Geometry: final body of the model. Coordinates: model frame, mm. A direction names the side the tool comes from. Give positions to 0.01 mm unless a question says otherwise; leave off trailing zeros. Order: outer loops, then holes, each group sorted by start corner. A loop starts at its lowest first (then second) coordinate and runs counter-clockwise, first axis right, second up. Notation, with made-up numbers: (1, -1) -> (40, -1) arc R21 ccw to (40, 28) -> close; hole circle Ø7 at (79.5, 32). An arc over 180 degrees is marked (long way). Answer in a Markdown table with one row per item. Add a question column.
Q1. Line query: line 1 along X through (y, z) = (20.5, -10.5); line 2 along Z through (x, y) = (-19, 11); line 3 along Y through (x, z) = (31, -78). Output: solid intervals per line, ascending. Write a range as from..to.
Q2. Set-up query: faces 1 (the face through (-99, 29.8, -10)), 2 (the face through (104, 20, -20)), 3 (the face through (-35.621, 5.029, -60.857)), 4 (the face through (1.92, 45.63, -87.48)), 5 (the face through (-104, 20, -20)). Return all of +Z, -Z, +X, -X, +Y, -Y with unobstructed straight access to the full face (end or side cutting, diameter ignored); none if empty.
Q3. Cut plane A-A on y = -11.5. Return the cut outline in (x, z), and give its area (3 significant figures).
Q4. Pull-direction query (Z, two-part tool) for faces 6 (the face through (-97, 64.8, -26)), 7 (the face through (99, 9.8, -10)), 8 (the face through (47.145, 1.496, -37.58)); classes: +Z half, -Z half, draft (parallel to the pull), parting line (faces both ways), or undercut.
Q5. Contact query for flat-ended pins moving along their axis: P1, Ø2, axis at x = -18.5, z = -18.5, coming from the -Y side; P2, Ø8, axis at y = -9, z = -77.5, coming from the -X side; P3, Ø4.5, axis at x = -96, z = -23, coming from the -Y side; P4, Ø3, axis at x = 46, y = 32.5, coming from the -Z side. Output: stop coordinate, or through.
from build123d import *
from build123d.topology import SkipClean

# Parameters (mm, degrees)
REVOLU_O2_ANGLE                     = 180
ESBO_O4_R                           = 10
RESSALTO_EXTRUS_O1_DEPTH            = 35
RESSALTO_EXTRUS_O2_DEPTH            = 20
ESBO_O6_R                           = 2.5
CORTE_EXTRUS_O1_DEPTH               = 15
ESBO_O9_R                           = 1.25
CORTE_EXTRUS_O3_DEPTH               = 6
RESSALTO_EXTRUS_O6_DEPTH            = 20
RESSALTO_EXTRUS_O7_DEPTH            = 20
CORTE_EXTRUS_O6_START               = 10
ESBO_O16_R                          = 93
CORTE_EXTRUS_O6_DEPTH               = 10
PADR_OCIRCULAR1_COUNT               = 2
PADR_OCIRCULAR1_ANGLE               = 60
PADR_OCIRCULAR1_THE_OTHER_WAY_COUNT = 2
PADR_OCIRCULAR1_THE_OTHER_WAY_ANGLE = 60
ESBO_O46_R                          = 3
CORTE_EXTRUS_O14_DEPTH              = 30
CORTE_EXTRUS_O15_DEPTH              = 175.966168158
CORTE_EXTRUS_O15_DEPTH_BACK         = 175.966168158


with BuildPart() as part:
    # Esboço3 → Revolução2 (revolve)
    with BuildSketch(Plane.XY):
        with BuildLine():
            Line((97.5, 79.8), (97.5, 11.304491341))
            Line((97.5, 11.304491341), (97.5, 0))
            Line((97.5, 0), (97.5, -40.2))
            Line((97.5, -40.2), (79.5, -40.2))
            Line((79.5, -40.2), (79.5, 0))
            Line((79.5, 0), (60.342408243, 0))
            Line((60.342408243, 0), (60.239391973, 2.95))
            Line((60.239391973, 2.95), (52, 2.95))
            Line((52, 2.95), (44, 10.95))
            Line((44, 10.95), (31, 10.95))
            Line((31, 10.95), (31, 13.7))
            Line((31, 13.7), (22.6, 13.7))
            Line((22.6, 13.7), (22.6, 17))
            Line((22.6, 17), (19.3, 17))
            Line((19.3, 17), (19.3, 17.7))
            Line((19.3, 17.7), (15.3, 17.7))
            Line((15.3, 17.7), (15.3, 21.05))
            Line((15.3, 21.05), (19.3, 21.05))
            Line((19.3, 21.05), (19.3, 21.2))
            Line((19.3, 21.2), (27.626549127, 25.96))
            Line((27.626549127, 25.96), (31.3, 25.96))
            Line((31.3, 25.96), (31.3, 43.96))
            Line((31.3, 43.96), (32.3, 44.96))
            Line((32.3, 44.96), (38.8, 44.96))
            Line((38.8, 44.96), (38.8, 26.9))
            Line((38.8, 26.9), (55.5, 10.2))
            Line((55.5, 10.2), (83.5, 10.2))
            ThreePointArc((83.5, 10.2), (86.328427125, 11.371572875), (87.5, 14.2))
            Line((87.5, 14.2), (87.5, 76.2))
            Line((87.5, 76.2), (93, 76.2))
            Line((93, 76.2), (93, 79.8))
            Line((93, 79.8), (97.5, 79.8))
        make_face()
    revolve(axis=Axis((0, -3.322055656, 0), (0, 1, 0)), revolution_arc=REVOLU_O2_ANGLE)

    # Esboço20 → Revolução3 (revolve)
    with SkipClean():  # the faces are left unmerged after this step: merging them gives an invalid solid
        with BuildSketch(Plane.XY, mode=Mode.PRIVATE) as revolu_o3_sk:
            Polygon((60.342408243, 2.95), (60.342408243, 10.2), (55.5, 10.2), (38.8, 26.9), (38.8, 44.96), (32.3, 44.96), (31.3, 43.96), (31.3, 25.96), (27.626549127, 25.96), (19.3, 21.2), (19.3, 21.05), (15.3, 21.05), (15.3, 17.7), (19.3, 17.7), (19.3, 17), (22.6, 17), (22.6, 13.7), (31, 13.7), (31, 10.95), (44, 10.95), (52, 2.95), align=None)
        revolve(revolu_o3_sk.sketch.rotate(Axis((0, -3.322055656, 0), (0, 1, 0)), 90), axis=Axis((0, -3.322055656, 0), (0, 1, 0)))
    add(part.part.scale(1), mode=Mode.REPLACE)  # the faces are merged on a copy

    # Esboço4 → Ressalto-extrusão1 (add)
    with BuildSketch(Plane(origin=(0, 79.8, 0), x_dir=(1, 0, 0), z_dir=(0, 1, 0))):
        with Locations((25.881656302, 96.591656302)):
            Circle(ESBO_O4_R)
        with Locations((-96.591656302, 25.881656302)):
            Circle(ESBO_O4_R)
    extrude(amount=-RESSALTO_EXTRUS_O1_DEPTH)

    # Esboço5 → Ressalto-extrusão2 (add)
    with BuildSketch(Plane.XZ.offset(40.2)):
        with BuildLine():
            Line((10, -105), (10, -96.985823706))
            Line((10, -96.985823706), (-10, -96.985823706))
            Line((-10, -96.985823706), (-10, -105))
            ThreePointArc((-10, -105), (0, -115), (10, -105))
        make_face()
    ressalto_extrus_o2 = extrude(amount=-RESSALTO_EXTRUS_O2_DEPTH)

    # Esboço6 → Corte-extrusão1 (cut)
    with BuildSketch(Plane(origin=(0, 79.8, 0), x_dir=(1, 0, 0), z_dir=(0, 1, 0))):
        with Locations(Location((25.881656302, 96.591656302, 0), (0, 0, 270))):
            Circle(ESBO_O6_R)
        with Locations(Location((-96.591656302, 25.881656302, 0), (0, 0, 270))):
            Circle(ESBO_O6_R)
    extrude(amount=-CORTE_EXTRUS_O1_DEPTH, mode=Mode.SUBTRACT)

    # Esboço9 → Corte-extrusão3 (cut)
    with BuildSketch(Plane.XZ.offset(-13.7)):
        with Locations(Location((18.738329701, -18.738329701, 0), (0, 0, 270))):
            Circle(ESBO_O9_R)
        with Locations(Location((-18.738329701, -18.738329701, 0), (0, 0, 270))):
            Circle(ESBO_O9_R)
        with Locations(Location((-18.738329701, 18.738329701, 0), (0, 0, 270))):
            Circle(ESBO_O9_R)
        with Locations(Location((18.738329701, 18.738329701, 0), (0, 0, 270))):
            Circle(ESBO_O9_R)
    extrude(amount=-CORTE_EXTRUS_O3_DEPTH, mode=Mode.SUBTRACT)

    # Esboço12 → Ressalto-extrusão6 (add)
    with BuildSketch(Plane.XY):
        with BuildLine():
            Line((-102, 29.8), (-87.5, 29.8))
            Line((-87.5, 29.8), (-87.5, 9.8))
            Line((-87.5, 9.8), (-102, 9.8))
            ThreePointArc((-102, 9.8), (-112, 19.8), (-102, 29.8))
        make_face()
    extrude(amount=-RESSALTO_EXTRUS_O6_DEPTH)

    # Esboço13 → Ressalto-extrusão7 (add)
    with BuildSketch(Plane.XY):
        with BuildLine():
            Line((102, 29.8), (93.1, 29.8))
            Line((93.1, 29.8), (93.1, 9.8))
            Line((93.1, 9.8), (102, 9.8))
            ThreePointArc((102, 9.8), (112, 19.8), (102, 29.8))
        make_face()
    extrude(amount=-RESSALTO_EXTRUS_O7_DEPTH)

    # Esboço16 → Corte-extrusão6 (cut)
    with BuildSketch(Plane(origin=(0, 76.2, 0), x_dir=(1, 0, 0), z_dir=(0, 1, 0)).offset(CORTE_EXTRUS_O6_START)):
        Circle(ESBO_O16_R)
    extrude(amount=-CORTE_EXTRUS_O6_DEPTH, mode=Mode.SUBTRACT)

    # PadrãoCircular1: Ressalto-extrusão2 ×2 about axis
    padr_ocircular1_axis = Axis((0, 0, 0), (0, 1, 0))
    for i in range(1, PADR_OCIRCULAR1_COUNT):
        add(ressalto_extrus_o2.rotate(padr_ocircular1_axis, i * PADR_OCIRCULAR1_ANGLE / (PADR_OCIRCULAR1_COUNT - 1)))

    # PadrãoCircular1 the other way: Ressalto-extrusão2 ×2 about axis
    padr_ocircular1_the_other_way_axis = Axis((0, 0, 0), (0, -1, 0))
    for i in range(1, PADR_OCIRCULAR1_THE_OTHER_WAY_COUNT):
        add(ressalto_extrus_o2.rotate(padr_ocircular1_the_other_way_axis, i * PADR_OCIRCULAR1_THE_OTHER_WAY_ANGLE / (PADR_OCIRCULAR1_THE_OTHER_WAY_COUNT - 1)))

    # Esboço46 → Corte-extrusão14 (cut)
    with BuildSketch(Plane(origin=(0, -20.2, 0), x_dir=(1, 0, 0), z_dir=(0, 1, 0))):
        with Locations(Location((90.932667397, 52.5, 0), (0, 0, 270))):
            Circle(ESBO_O46_R)
        with Locations(Location((0, 105, 0), (0, 0, 270))):
            Circle(ESBO_O46_R)
        with Locations(Location((-90.932667397, 52.5, 0), (0, 0, 270))):
            Circle(ESBO_O46_R)
    extrude(amount=-CORTE_EXTRUS_O14_DEPTH, mode=Mode.SUBTRACT)

    # Esboço47 → Corte-extrusão15 (cut, two sides: drawn at the far end of the back side and taken through both)
    with SkipClean():  # the faces are left unmerged after this step: merging them gives an invalid solid
        with BuildSketch(Plane(origin=(0, 10.2, 0), x_dir=(1, 0, 0), z_dir=(0, 1, 0)).offset(-CORTE_EXTRUS_O15_DEPTH_BACK)):
            with BuildLine():
                Line((-60.827262138, 45.377960052), (-9.698115338, 76.775576961))
                ThreePointArc((-9.698115338, 76.775576961), (11.156996709, 71.489405367), (5.307399574, 50.785262738))
                Line((5.307399574, 50.785262738), (-45.821747226, 19.38764583))
                ThreePointArc((-45.821747226, 19.38764583), (-66.676859273, 24.673817424), (-60.827262138, 45.377960052))
            make_face()
        extrude(amount=CORTE_EXTRUS_O15_DEPTH + CORTE_EXTRUS_O15_DEPTH_BACK, mode=Mode.SUBTRACT)


solid = part.part
Completed:
| question | item | result |
|---|---|---|
| 1 | line 1 | x = -111.98..-86.87, -43.96..-11.13, 11.13..43.96, 86.87..111.98 |
| 1 | line 2 | z = -95.63..-83.77, -35.86..-24.49, 24.49..51.29 |
| 1 | line 3 | y = -40.2..10.22 |
| 2 | face 1 | -Z, -X |
| 2 | face 2 | -Z, +X, +Y, -Y |
| 2 | face 3 | +Y, -Y |
| 2 | face 4 | +Y |
| 2 | face 5 | -Z, -X, -Y |
| 3 | outline | (-97.5, 0) arc R97.5 ccw to (97.5, 0) -> (79.5, 0) arc R79.5 cw to (-79.5, 0) -> close |
| 3 | area | 5,000 mm² |
| 4 | face 6 | undercut |
| 4 | face 7 | draft |
| 4 | face 8 | +Z half |
| 5 | P1 | stops at y = 13.7 |
| 5 | P2 | stops at x = -64.06 |
| 5 | P3 | stops at y = -40.2 |
| 5 | P4 | stops at z = -86.75 |
